from build123d import *

# Parameters (mm, degrees)
BOSS_EXTRUDE1_DEPTH = 15
SKETCH2_R           = 1.75
CUT_EXTRUDE1_DEPTH  = 15


with BuildPart() as part:
    # Sketch1 → Boss-Extrude1 (new body)
    with BuildSketch(Plane(origin=(0, 0, 0), x_dir=(1, 0, 0), z_dir=(0, 1, 0))):
        with BuildLine():
            Line((12.4, 5.1), (12.6, 0))
            Line((12.6, 0), (22.6, 0))
            Line((22.6, 0), (22.6, 2))
            Line((22.6, 2), (14.6, 2))
            Line((14.6, 2), (14.6, 11.6))
            Line((14.6, 11.6), (-2, 11.6))
            Line((-2, 11.6), (-2, 2))
            Line((-2, 2), (-10, 2))
            Line((-10, 2), (-10, 0))
            Line((-10, 0), (0, 0))
            Line((0, 0), (0.2, 0))
            Line((0.2, 0), (0.2, 5.1))
            add(Edge.make_bspline(
                [(2.3, 9.6), (0.2, 7.65), (0.2, 5.1)],
                knots=[0, 0, 0, 0.5, 0.5, 0.5], degree=2))
            Line((2.3, 9.6), (10.3, 9.6))
            add(Edge.make_bspline(
                [(10.3, 9.6), (12.4, 7.65), (12.4, 5.1)],
                knots=[0, 0, 0, 0.5, 0.5, 0.5], degree=2))
        make_face()
    extrude(amount=BOSS_EXTRUDE1_DEPTH)

    # Sketch2 → Cut-Extrude1 (cut)
    with BuildSketch(Plane(origin=(0, 0, -2), x_dir=(-1, 0, 0), z_dir=(0, 0, -1))):
        with Locations((-18.6, 7.5)):
            Circle(SKETCH2_R)
        with Locations((6, 7.5)):
            Circle(SKETCH2_R)
    extrude(amount=-CUT_EXTRUDE1_DEPTH, mode=Mode.SUBTRACT)


solid = part.part
Design review of the part built by this model. Coordinates are the model's own, in mm. A direction names the side the tool comes from. Give positions to 0.01 mm unless a question says otherwise; leave off trailing zeros. Write each loop counter-clockwise with the first axis right and the second up, starting at its lowest first coordinate (ties: lowest second). Pieces come first, ordered by that corner, then holes. Notation, with made-up numbers: M 26.5,10.25 L 79.5,10.25 A24 cw 79.5,44.25 Z; hole C 34,18 d9. An arc over 180 degrees is marked long. Answer as a JSON object with one key per item and string values. Group by question number.
1) Clearance check with flat-ended pins moving along their axes: pin 1 Ø2 at (x, z) = (16.5, -5) entering from +Y; pin 2 Ø4 at (x, y) = (-5, 9) entering from -Z; pin 3 Ø5 at (y, z) = (9.5, -9) entering from +X; pin 4 Ø5 at (y, z) = (7.5, -6) entering from -X. State where each tip first meets the part, or that it passes through.
2) We need section C-C (y = 7.5). Count the separate pieces of the cut face and the enclosed holes in it, and give its area (3 significant figures).
3) We need section B-B (z = -1). Give the boundary of the cut face in (x, y).
4) For line 1 along Y through (x, z) = (18.6, -0.65); line 2 along X through (y, z) = (13.75, -3.25); line 3 along Z through (x, y) = (10, 6.5), list the stretches that pass through material, from the lowest coordinate up.
5) We need section A-A (x = -6). Give the boundary of the cut face in (y, z).
6) Tool access review of faces 1 (the face through (-4, 7, -2)), 2 (the face through (-5.62, 5.79, -1.01)), 3 (the face through (22.6, 7, -1)), 4 (the face through (20, 6, -2)), 5 (the face through (12.5, 7.4, -2.6)): name each direction out of +Z, -Z, +X, -X, +Y, -Y from which nothing blocks a thin tool from reaching the whole face with its end or side.
7) Mouldability with a two-part tool opening along Y and no side actions: class faces 6 (the face through (19.99, 6.44, -1.01)), 7 (the face through (6, 0, -10)), 8 (the face through (6, 15, -10)), 9 (the face through (14.6, 7, -7)) as released by +Y, released by -Y, zero draft, split by the parting line, or undercut.
8) We need section D-D (z = -3.75). Give the boundary of the cut face in (x, y), and give its area (3 significant figures).
Answer key:
{
 "1": {"pin 1": "passes through", "pin 2": "stops at z = -2", "pin 3": "stops at x = 14.6", "pin 4": "stops at x = -2"},
 "2": {"separate pieces": "3", "enclosed holes": "0", "area": "98.8 mm²"},
 "3": {"outline": "M -10,0 L 0.2,0 L 0.2,15 L -10,15 Z; M 12.56,0 L 22.6,0 L 22.6,15 L 12.56,15 Z; hole C -6,7.5 d3.5; hole C 18.6,7.5 d3.5"},
 "4": {"line 1": "y = 0 to 5.75, 9.25 to 15", "line 2": "x = -2 to 0.2, 12.47 to 14.6", "line 3": "z = -11.6 to -9.6"},
 "5": {"outline": "M 0,-2 L 5.75,-2 L 5.75,0 L 0,0 Z; M 9.25,-2 L 15,-2 L 15,0 L 9.25,0 Z"},
 "6": {"face 1": "-Z, -X, +Y, -Y", "face 2": "+Z, -Z", "face 3": "+Z, -Z, +X, +Y, -Y", "face 4": "-Z, +X, +Y, -Y", "face 5": "+Z, +Y, -Y"},
 "7": {"face 6": "undercut", "face 7": "released by -Y", "face 8": "released by +Y", "face 9": "zero draft"},
 "8": {"outline": "M -2,0 L 0.2,0 L 0.2,15 L -2,15 Z; M 12.45,0 L 14.6,0 L 14.6,15 L 12.45,15 Z", "area": "65.2 mm²"}
}
